Model file for the job. Use its own axes, mm. Face numbers are marked on the shaded views. A direction names the side the tool comes from. Round coordinates to 2 decimals unless told otherwise and drop trailing zeros. Order: outer loops, then holes, each group sorted by start corner. A loop starts at its lowest first (then second) coordinate and runs counter-clockwise, first axis right, second up. Notation, with made-up numbers: (50.25, 46) -> (97.25, 46) arc R20 cw to (97.25, 57) -> close; hole circle Ø9 at (-12, -4.75). An arc over 180 degrees is marked (long way). Put each result on its own line as item: value. Start each with the question number.
Q1. Probe L1, parallel to X at y = -33.5, z = 1; L2, parallel to X at y = 22, z = 2.75. List the from-to ranges inside material, lowest first.
Q2. Cut at B-B, the plane y = -16.5. List the corners of the cut face in (x, z), and give its area (3 significant figures).
Q3. Cut at D-D, the plane x = 6.75. List the corners of the cut face in (y, z).
Q4. Pull direction X, two halves, no side cores. Call the marked faces 3, 4 and 5: released by +X, released by -X, zero draft, split by the parting line, or undercut.
Q5. Flat gauge pins, fed straight in: P1, Ø1, axis at x = 33, y = -33, coming from the +Z side; P2, Ø10, axis at x = -6, y = 1.5, coming from the +Z side. Where does each tip first touch, or does it go through?
Q6. 3-axis set-ups, long thin cutter, end or side, ignore diameter. For the marked faces 1 and 2: which of +Z, -Z, +X, -X, +Y, -Y reach the whole face in a straight line?
Q7. Cut at A-A, the plane z = 6.25. List the corners of the cut face in (x, y), and give its area (3 significant figures).
Autodesk Inventor part; units mm, degrees
ref_plane "YZ Plane" through (0, 0, 0) normal (1, 0, 0) x (0, 1, 0)
ref_plane "XZ Plane" through (0, 0, 0) normal (0, 1, 0) x (-1, 0, 0)
ref_plane "XY Plane" through (0, 0, 0) normal (0, 0, 1) x (1, 0, 0)
sketch "USB_Micro" plane through (0, 0, 0) normal (0, 0, 1) x (1, 0, 0)
  line L0 (-6.7, 3.4) -> (-6.7, 2.0438)
  line L1 (-7.2, 1.6938) -> (-6.7, 2.0438)
  line L2 (-7.2, 1.6938) -> (-7.2, 0.3)
  line L3 (-7.2, 0.3) -> (-0.3, 0.3)
  line L4 (-0.3, 0.3) -> (-0.3, 1.6938)
  line L5 (-0.8, 2.0438) -> (-0.3, 1.6938)
  line L6 (-6.7, 3.4) -> (-0.8, 3.4)
  line L7 (-0.8, 3.4) -> (-0.8, 2.0438)
  line L8 (-0.8, 0.8) -> (-6.7, 0.8)
  line L9 (-6.7, 0.8) -> (-6.7, 1.4335)
  line L10 (-6.7, 1.4335) -> (-6.2, 1.7835)
  line L11 (-6.2, 1.7835) -> (-6.2, 2.9)
  line L12 (-6.2, 2.9) -> (-1.3, 2.9)
  line L13 (-1.3, 2.9) -> (-1.3, 1.7835)
  line L14 (-1.3, 1.7835) -> (-0.8, 1.4335)
  line L15 (-0.8, 1.4335) -> (-0.8, 0.8)
  point P0 (-3.75, 0.3)
  dimension "d42" = 0.5
sketch "Skizze1" plane through (0, 0, 0) normal (0, 0, 1) x (1, 0, 0)
  line L0 (-39, -39) -> (39, -39)
  line L1 (39, -39) -> (39, 39)
  line L2 (39, 39) -> (-39, 39)
  line L3 (-39, 39) -> (-39, -39)
  line L4 (-39, -39) -> (39, 39) construction
  line L5 (39, -39) -> (-39, 39) construction
  line L6 (-37.5, -37.5) -> (37.5, -37.5)
  line L7 (37.5, -37.5) -> (37.5, 37.5)
  line L8 (37.5, 37.5) -> (-37.5, 37.5)
  line L9 (-37.5, 37.5) -> (-37.5, -37.5)
  line L10 (-37.5, -37.5) -> (37.5, 37.5) construction
  line L11 (37.5, -37.5) -> (-37.5, 37.5) construction
  line L12 (-37.5, 37.5) -> (-35.5, 37.5)
  line L13 (-35.5, 37.5) -> (-35.5, -37.5)
  line L14 (-35.5, -37.5) -> (-37.5, -37.5)
  line L15 (-37.5, -37.5) -> (-37.5, 37.5)
  line L16 (35.5, 37.5) -> (37.5, 37.5)
  line L17 (37.5, 37.5) -> (37.5, -37.5)
  line L18 (37.5, -37.5) -> (35.5, -37.5)
  line L19 (35.5, -37.5) -> (35.5, 37.5)
  line L20 (-35.5, -35.5) -> (35.5, -35.5)
  line L21 (35.5, -35.5) -> (35.5, -37.5)
  line L22 (35.5, -37.5) -> (-35.5, -37.5)
  line L23 (-35.5, -37.5) -> (-35.5, -35.5)
  line L24 (35.5, 37.5) -> (-35.5, 37.5)
  line L25 (-35.5, 37.5) -> (-35.5, 35.5)
  line L26 (-35.5, 35.5) -> (35.5, 35.5)
  line L27 (35.5, 35.5) -> (35.5, 37.5)
  point P0 (0, 0)
  dimension "d0" = 78
  dimension "d1" = 78
  dimension "d2" = 75
  dimension "d3" = 75
  dimension "d46" = 2
  dimension "d47" = 2
  dimension "d48" = 2
  dimension "d52" = 2
extrude "Extrusion1" add sketch "Skizze1" along normal blind 15
extrude "Extrusion9" add sketch "Skizze1" along normal blind 5 contours L9 L8 L13 L6 | L13 L20 L19 L6 | L19 L8 L7 L6 | L8 L19 L26 L13
extrude "Extrusion6" add sketch "Skizze1" against normal blind 2 contours L3 L2 L1 L0 | L9 L8 L13 L6 | L13 L20 L19 L6 | L19 L8 L7 L6 | L13 L26 L19 L20 | L8 L19 L26 L13
sketch "Skizze5" plane through (0, 0, 0) normal (0, 0, 1) x (1, 0, 0)
  circle A0 centre (32.75, -32.75) radius 1
  circle A1 centre (32.75, 32.75) radius 1
  circle A2 centre (6.75, -32.75) radius 1
  circle A3 centre (6.75, 32.75) radius 1
  circle A4 centre (32.75, 32.75) radius 2.5
  circle A5 centre (6.75, 32.75) radius 2.5
  circle A6 centre (32.75, -32.75) radius 2.5
  circle A7 centre (6.75, -32.75) radius 2.5
  line L0 (-54.6, 0) -> (54.6, 0)
  line L1 (0, -54.6) -> (0, 54.6)
  line L2 (35.5, 35.5) -> (35.5, -35.5)
  line L3 (-35.5, 35.5) -> (35.5, 35.5)
  line L4 (35.5, -35.5) -> (-35.5, -35.5)
  line L5 (9.25, 32.75) -> (9.25, 35.5)
  line L6 (4.25, 32.75) -> (4.25, 35.5)
  line L7 (4.25, 35.5) -> (9.25, 35.5)
  line L8 (30.25, 32.75) -> (30.25, 35.5)
  line L9 (30.25, 35.5) -> (35.5, 35.5)
  line L10 (32.75, 30.25) -> (35.5, 30.25)
  line L11 (35.5, 30.25) -> (35.5, 35.5)
  line L12 (32.75, -30.25) -> (35.5, -30.25)
  line L13 (35.5, -30.25) -> (35.5, -35.5)
  line L14 (30.25, -32.75) -> (30.25, -35.5)
  line L15 (30.25, -35.5) -> (35.5, -35.5)
  line L16 (9.25, -32.75) -> (9.25, -35.5)
  line L17 (4.25, -32.75) -> (4.25, -35.5)
  line L18 (4.25, -35.5) -> (9.25, -35.5)
  point P0 (0, 0)
  dimension "d28" = 2
  dimension "d33" = 5
  dimension "d34" = 65.5
  dimension "d35" = 26
  dimension "d36" = 32.75
  dimension "d37" = 32.75
  dimension "d51" = 32.75
extrude "Extrusion7" add sketch "Skizze5" along normal blind 4 contours A4 | A5 | A6 | A7
sketch "Skizze6" plane through (-39, 39, 15) normal (0, 1, 0) x (1, 0, 0)
  line L0 (63.71, 5.7) -> (56.21, 5.7)
  line L1 (63.71, 7.55) -> (63.71, 5.7)
  line L2 (63.71, 7.55) -> (63.21, 7.9)
  line L3 (63.21, 7.9) -> (63.21, 9.4)
  line L4 (56.71, 9.4) -> (63.21, 9.4)
  line L5 (56.71, 7.9) -> (56.71, 9.4)
  line L6 (56.21, 7.55) -> (56.71, 7.9)
  line L7 (56.21, 7.55) -> (56.21, 5.7)
  line L8 (56.51, 6) -> (63.41, 6)
  line L9 (56.51, 7.3938) -> (56.51, 6)
  line L10 (57.01, 7.7438) -> (56.51, 7.3938)
  line L11 (57.01, 9.1) -> (57.01, 7.7438)
  line L12 (62.91, 9.1) -> (57.01, 9.1)
  line L13 (62.91, 9.1) -> (62.91, 7.7438)
  line L14 (62.91, 7.7438) -> (63.41, 7.3938)
  line L15 (63.41, 7.3938) -> (63.41, 6)
  line L16 (64.46, 4.95) -> (55.46, 4.95)
  line L17 (55.46, 4.95) -> (55.46, 7.9405)
  line L18 (55.46, 7.9405) -> (55.96, 8.2905)
  line L19 (55.96, 8.2905) -> (55.96, 10.15)
  line L20 (55.96, 10.15) -> (63.96, 10.15)
  line L21 (63.96, 10.15) -> (63.96, 8.2905)
  line L22 (63.96, 8.2905) -> (64.46, 7.9405)
  line L23 (64.46, 7.9405) -> (64.46, 4.95)
  point P0 (39, 15)
  dimension "d45" = 0.75
extrude "Extrusion8" [suppressed]
extrude "Extrusion10" add sketch "Skizze5" along normal blind 8 contours A0 | A1 | A2 | A3
extrude "Extrusion11" add sketch "Skizze5" along normal up to surface (4 mm away) contours A4 L8 L3 L2 L10 | L5 A5 L6 L3 | L2 L4 L14 A6 L12 | L17 A7 L16 L4
sketch "Skizze7" plane through (-39, 39, 15) normal (0, 1, 0) x (1, 0, 0)
  line L0 (78, 0) -> (0, 0)
  line L1 (78, 17) -> (78, 0)
  line L2 (61.25, 0) -> (61.25, 2.5)
  line L3 (56.25, 2.5) -> (56.25, 0)
  line L4 (1.5, 0) -> (76.5, 0)
  line L5 (61.25, 0) -> (56.25, 0)
  arc A0 (61.25, 2.5) -> (56.25, 2.5) centre (58.75, 2.5) ccw
  point P0 (39, 15)
  dimension "d58" = 19.25
  dimension "d59" = 5
  dimension "d60" = 2.5
extrude "Extrusion12" cut sketch "Skizze7" against normal up to surface (1.5 mm away)
equation "\"d0\" = d1"
equation "\"d2\" = d3"
equation "\"d47\" = d46"
equation "\"d48\" = d46"
equation "\"d52\" = d46"
properties part number "Sensorlamp_Base_new"
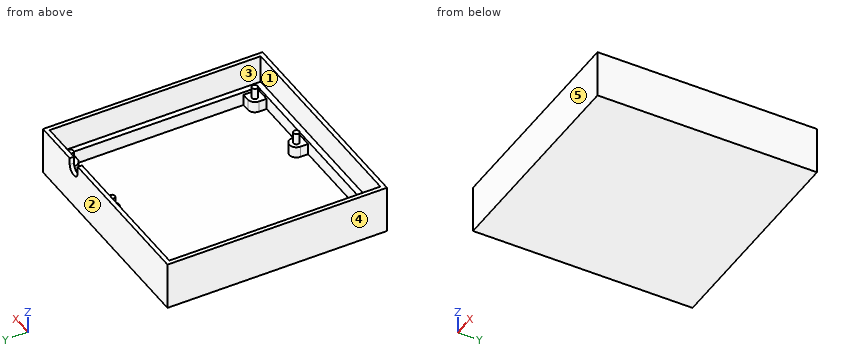
Ans:
1. L1: x = -39 to -35.5, 4.25 to 9.25, 30.25 to 39
1. L2: x = -39 to -35.5, 35.5 to 39
2. outline: (-39, -2) -> (39, -2) -> (39, 15) -> (37.5, 15) -> (37.5, 5) -> (35.5, 5) -> (35.5, 0) -> (-35.5, 0) -> (-35.5, 5) -> (-37.5, 5) -> (-37.5, 15) -> (-39, 15) -> close
2. area: 221 mm^2
3. outline: (-39, -2) -> (39, -2) -> (39, 15) -> (37.5, 15) -> (37.5, 5) -> (35.5, 5) -> (35.5, 4) -> (33.75, 4) -> (33.75, 8) -> (31.75, 8) -> (31.75, 4) -> (30.25, 4) -> (30.25, 0) -> (-30.25, 0) -> (-30.25, 4) -> (-31.75, 4) -> (-31.75, 8) -> (-33.75, 8) -> (-33.75, 4) -> (-35.5, 4) -> (-35.5, 5) -> (-37.5, 5) -> (-37.5, 15) -> (-39, 15) -> close
4. face 3: undercut
4. face 4: released by -X
4. face 5: zero draft
5. P1: stops at z = 8
5. P2: stops at z = 0
6. face 1: +Z
6. face 2: +Z, -Z, +X, -X, +Y
7. outline: (-39, -39) -> (39, -39) -> (39, 39) -> (-39, 39) -> close; circle Ø2 at (6.75, -32.75); circle Ø2 at (6.75, 32.75); circle Ø2 at (32.75, -32.75); circle Ø2 at (32.75, 32.75); hole (-37.5, -37.5) -> (37.5, -37.5) -> (37.5, 37.5) -> (-37.5, 37.5) -> close
7. area: 472 mm^2
